The listing builds one solid part. Answer for the finished solid, in the listing's coordinates (mm). A direction names the side the tool comes from. Round coordinates to 2 decimals unless told otherwise and drop trailing zeros. Write each loop counter-clockwise with the first axis right and the second up, starting at its lowest first coordinate (ties: lowest second). Pieces come first, ordered by that corner, then holes.
Item 1: Find section A-A on z = -66.04. Give the vertices of the cut face in (x, y).
Item 2: A tool of negligible diameter and unlimited length cuts with its end or side. For faces 4 (the face through (-27, -2, -78.58)), 5 (the face through (-27, -12, -73.58)), 6 (the face through (-27, -10, 10)), 7 (the face through (-27, -22, -93.58)), 8 (the face through (-27, -25, 8)), from which of +Z, -Z, +X, -X, +Y, -Y can it reach the whole face along a straight path? Write none if from no direction.
Item 3: Find section B-B on y = -1.5. Give the vertices of the cut face in (x, z), then the cut area to 3 significant figures.
Item 4: Find section C-C on z = -41.5. Give the vertices of the cut face in (x, y), then the cut area to 3 significant figures.
Item 5: For a pull along X with two mould halves and no side action, classify faces 1 (the face through (-26, -25, -91)), 2 (the face through (-7, 2.5, -67.5)), 3 (the face through (10, 1, -54)) as +X half, -X half, draft (parallel to the pull), parting line (faces both ways), or undercut.
Item 6: Each of these flat-tipped pins is pushed along its axis until it touches: pin 1 (10 mm diameter, centred on x = -18.5, y = -3, fed in from -Z); pin 2 (5.5 mm diameter, centred on x = -25, y = -23, fed in from -Z); pin 3 (4 mm diameter, centred on x = -35.56, z = -66.04, fed in from -Y); pin 4 (17 mm diameter, centred on x = -12, z = -99.5, fed in from +Y). Where does it stop, or does it pass through?
Item 7: Find the intervals of material crossed by probe 1 along Z at (x, y) = (3.5, -4); probe 2 along X at (y, z) = (3.3, -66.04); probe 3 along X at (y, z) = (3.8, -15.24), in increasing order.
```python
from build123d import *

# Parameters (mm, degrees)
SKETCH2_W           = 73.34
SKETCH2_H           = 88.58
BOSS_EXTRUDE1_DEPTH = 5
SKETCH1_R           = 1.5875
CUT_EXTRUDE3_DEPTH  = 50
SKETCH3_W           = 73.34
SKETCH3_H           = 5
BOSS_EXTRUDE2_DEPTH = 25
SKETCH4_W           = 73.34
SKETCH4_H           = 5
BOSS_EXTRUDE3_DEPTH = 40
CUT_EXTRUDE4_DEPTH  = 40
VARFILLET1_START    = -64
VARFILLET1_DEPTH    = 75
VARFILLET2_START    = -63.34
VARFILLET2_DEPTH    = 73.34


with BuildPart() as part:
    # Sketch2 → Boss-Extrude1 (new body)
    with BuildSketch(Plane(origin=(0, 0, 0), x_dir=(1, 0, 0), z_dir=(0, 1, 0))):
        with Locations((-26.67, 34.29)):
            Rectangle(SKETCH2_W, SKETCH2_H)
    extrude(amount=BOSS_EXTRUDE1_DEPTH)

    # Sketch1 → Cut-Extrude3 (cut)
    with BuildSketch(Plane(origin=(0, 0, 0), x_dir=(1, 0, 0), z_dir=(0, 1, 0))):
        with Locations(Location((-7.62, 66.04, 0), (0, 0, 90))):
            Circle(SKETCH1_R)
        with Locations(Location((-35.56, 66.04, 0), (0, 0, 90))):
            Circle(SKETCH1_R)
        with Locations(Location((-2.54, 13.97, 0), (0, 0, 90))):
            Circle(SKETCH1_R)
        with Locations(Location((-50.8, 15.24, 0), (0, 0, 90))):
            Circle(SKETCH1_R)
    extrude(amount=CUT_EXTRUDE3_DEPTH, mode=Mode.SUBTRACT)

    # Sketch3 → Boss-Extrude2 (add)
    with BuildSketch(Plane.XZ):
        with Locations((-26.67, -76.08)):
            Rectangle(SKETCH3_W, SKETCH3_H)
        with Locations((-26.67, 7.5)):
            Rectangle(SKETCH3_W, SKETCH3_H)
    extrude(amount=BOSS_EXTRUDE2_DEPTH)

    # Sketch4 → Boss-Extrude3 (add)
    with BuildSketch(Plane(origin=(0, 0, -78.58), x_dir=(-1, 0, 0), z_dir=(0, 0, -1))):
        with Locations((26.67, -22.5)):
            Rectangle(SKETCH4_W, SKETCH4_H)
    extrude(amount=BOSS_EXTRUDE3_DEPTH)

    # Sketch5 → Cut-Extrude4 (cut)
    with BuildSketch(Plane(origin=(0, -20, 0), x_dir=(1, 0, 0), z_dir=(0, 1, 0))):
        with BuildLine():
            Line((-41.67, 93.58), (-11.67, 93.58))
            ThreePointArc((-11.67, 93.58), (-6.67, 98.58), (-11.67, 103.58))
            Line((-11.67, 103.58), (-41.67, 103.58))
            ThreePointArc((-41.67, 103.58), (-46.67, 98.58), (-41.67, 93.58))
        make_face()
    extrude(amount=-CUT_EXTRUDE4_DEPTH, mode=Mode.SUBTRACT)

    # VarFillet1: read off the stored shape, not the designer's step
    # VarFillet1 outline → VarFillet1 (cut)
    with BuildSketch(Plane.YZ.offset(VARFILLET1_START)):
        with BuildLine():
            add(Edge.make_bspline(
                [(-25, -118.58), (-20, -115.693248654), (-20, -109.919745962)],
                knots=[0, 0, 0, 1, 1, 1], degree=2, weights=[1, 0.866025404, 1]))
            Line((-25, -118.58), (-20, -118.58))
            Line((-20, -118.58), (-20, -109.919745962))
        make_face()
    extrude(amount=VARFILLET1_DEPTH, mode=Mode.SUBTRACT)

    # VarFillet2: read off the stored shape, not the designer's step
    # VarFillet2 outline → VarFillet2 (add)
    with BuildSketch(Plane.YZ.offset(VARFILLET2_START)):
        with BuildLine():
            Line((-20, -78.58), (-20, -88.58))
            add(Edge.make_bspline(
                [(-20, -88.58), (-20, -78.58), (-10, -78.58)],
                knots=[0, 0, 0, 1, 1, 1], degree=2, weights=[1, 0.707106781, 1]))
            Line((-10, -78.58), (-20, -78.58))
        make_face()
    extrude(amount=VARFILLET2_DEPTH)


solid = part.part
```
Check values:
1. outline: (-63.34, 0) - (-37.15, 0) - (-37.15, 5) - (-63.34, 5) - close; (-33.97, 0) - (-9.21, 0) - (-9.21, 5) - (-33.97, 5) - close; (-6.03, 0) - (10, 0) - (10, 5) - (-6.03, 5) - close
2. face 4: -Z, +X, -X, +Y
2. face 5: +X, -X, -Y
2. face 6: +Z, +X, -X, +Y, -Y
2. face 7: +Y, -Y
2. face 8: +Z, -Z, +X, -X, -Y
3. outline: (-63.34, -78.58) - (10, -78.58) - (10, -73.58) - (-63.34, -73.58) - close; (-63.34, 5) - (10, 5) - (10, 10) - (-63.34, 10) - close
3. area: 733 mm2
4. outline: (-63.34, 0) - (10, 0) - (10, 5) - (-63.34, 5) - close
4. area: 367 mm2
5. face 1: draft
5. face 2: undercut
5. face 3: +X half
6. pin 1: stops at z = -78.58
6. pin 2: stops at z = -118.58
6. pin 3: stops at y = 0
6. pin 4: stops at y = -20
7. probe 1: z = -78.58 to -73.58, 5 to 10
7. probe 2: x = -63.34 to -37.15, -33.97 to -9.21, -6.03 to 10
7. probe 3: x = -63.34 to -52.39, -49.21 to -3.49, -1.59 to 10
